Design review of the part built by this model. Coordinates are the model's own, in mm. A direction names the side the tool comes from. Round coordinates to 2 decimals unless told otherwise and drop trailing zeros. Order: outer loops, then holes, each group sorted by start corner. A loop starts at its lowest first (then second) coordinate and runs counter-clockwise, first axis right, second up. Notation, with made-up numbers: M 10,86.5 L 40,86.5 A21 ccw 40,105.5 Z; hole C -17.5,87 d7. An arc over 180 degrees is marked long. Use a Markdown table: item, result. Add a question column.
(1) Take a section at A-A (x = -7.5). Write out the cut boundary in (y, z).
(2) For pin 1 (2.5 mm diameter, centred on y = 2, z = -10, fed in from +X); pin 2 (5 mm diameter, centred on x = -9.5, z = 11.5, fed in from +Y); pin 3 (1.6 mm diameter, centred on x = 2.5, y = 6, fed in from +Z), all flat-tipped, find the tip position at first contact; note any pin that passes through.
(3) Take a section at B-B (z = 1.5). Write out the cut boundary in (x, y).
(4) Machinability: for faces 1 (the face through (0, 6, 7.5)), 2 (the face through (-9.226, 6, 4)), 3 (the face through (0, 2, -10)), 4 (the face through (0, 7, 4)), 5 (the face through (9.226, 6, 4)), which of the approach directions +Z, -Z, +X, -X, +Y, -Y give a long, thin tool a straight path to every point of the face, cutting with its end or side? Answer none if there is none.
(5) Take a section at C-C (x = 2.25). Write out the cut boundary in (y, z), then the cut area to 3 significant figures.
(6) To check wall thickness, follow probe 1 along X at (y, z) = (1, -5); probe 2 along Z at (x, y) = (4, 6.75); probe 3 along Z at (x, y) = (7.5, 3.75). State the ranges of each line that lie inside material, in increasing order. Write a range as from..to.
(7) Take a section at D-D (z = -3.5). Write out the cut boundary in (x, y).
```python
from build123d import *

# Parameters (mm, degrees)
BOSS_EXTRUDE1_DEPTH = 5
CUT_EXTRUDE1_REACH  = 7
SKETCH3_W           = 18.452994616
SKETCH3_H           = 7.5
BOSS_EXTRUDE2_DEPTH = 2


with BuildPart() as part:
    # Sketch1 → Boss-Extrude1 (new body)
    with BuildSketch(Plane(origin=(0, 0, 0), x_dir=(1, 0, 0), z_dir=(0, 1, 0))):
        Polygon((0, 0), (0, 20), (-25, 20), (-25, -20), (-8.000491869, -49.444011787), (8.000491869, -49.444011787), (25, -20), (25, 0), align=None)
    extrude(amount=BOSS_EXTRUDE1_DEPTH)

    # Sketch2 → Cut-Extrude1 (cut, up to next)
    with BuildSketch(Plane(origin=(0, 5, 0), x_dir=(1, 0, 0), z_dir=(0, 1, 0)), mode=Mode.PRIVATE) as cut_extrude1_sk1:
        Polygon((-15, 20), (-15, -5), (-9.226497308, -15), (9.226497308, -15), (15, -5), (15, 0), (25, 0), (25, -20), (8.000491869, -49.444011787), (-8.000491869, -49.444011787), (-25, -20), (-25, 20), align=None)
    cut_extrude1_tool1 = extrude(cut_extrude1_sk1.sketch, amount=-CUT_EXTRUDE1_REACH, mode=Mode.PRIVATE) & part.part
    add(cut_extrude1_tool1.solids().sort_by_distance((-2.247946, 5, 20.557757))[0], mode=Mode.SUBTRACT)

    # Sketch3 → Boss-Extrude2 (add)
    with BuildSketch(Plane(origin=(0, 5, 0), x_dir=(1, 0, 0), z_dir=(0, 1, 0))):
        with Locations((0, -3.75)):
            Rectangle(SKETCH3_W, SKETCH3_H)
    extrude(amount=BOSS_EXTRUDE2_DEPTH)


solid = part.part
```
Verdict:
| question | item | result |
|---|---|---|
| 1 | outline | M 0,-20 L 5,-20 L 5,0 L 7,0 L 7,7.5 L 5,7.5 L 5,15 L 0,15 Z |
| 2 | pin 1 | stops at x = 0 |
| 2 | pin 2 | stops at y = 5 |
| 2 | pin 3 | stops at z = 7.5 |
| 3 | outline | M -15,0 L 15,0 L 15,5 L 9.23,5 L 9.23,7 L -9.23,7 L -9.23,5 L -15,5 Z |
| 4 | face 1 | +Z, +X, -X, +Y |
| 4 | face 2 | +Z, -Z, -X, +Y |
| 4 | face 3 | -Z, +X, +Y, -Y |
| 4 | face 4 | +Z, -Z, +X, -X, +Y |
| 4 | face 5 | +Z, -Z, +X, +Y |
| 5 | outline | M 0,0 L 7,0 L 7,7.5 L 5,7.5 L 5,15 L 0,15 Z |
| 5 | area | 90.0 mm^2 |
| 6 | probe 1 | x = -15..0 |
| 6 | probe 2 | z = 0..7.5 |
| 6 | probe 3 | z = 0..15 |
| 7 | outline | M -15,0 L 0,0 L 0,5 L -15,5 Z |
